Study the drawing (mm; zero at the part's minimum x, y, z) and answer. A direction names the side the tool comes from. Round coordinates to 2 decimals unless told otherwise and drop trailing zeros. Write each loop counter-clockwise with the first axis right and the second up, starting at its lowest first coordinate (ties: lowest second). Pieces come first, ordered by that corner, then holes. Notation, with made-up numbers: (-30, 73) -> (-5, 73) arc R18 cw to (-5, 108) -> close; hole circle Ø7 at (22.25, -30.75). An arc over 180 degrees is marked (long way). Return JSON: item names as keys, results as strings.
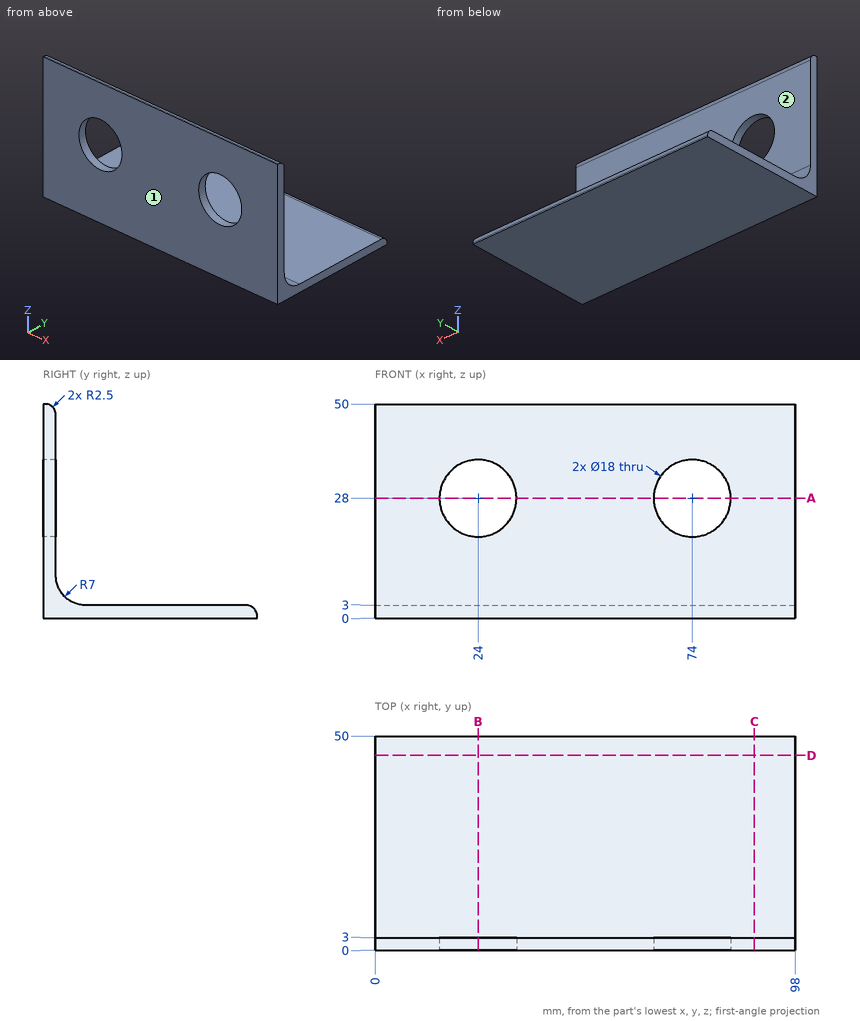
Item 1: Section D-D (y = 45.5) is taken. Give the vertices of the cut face in (x, z), then the cut area to 3 significant figures.
Worked answers:
{"outline": "(0, 0) -> (98, 0) -> (98, 3) -> (0, 3) -> close", "area": "294 mm2"}
Item 2: A tool of negligible diameter and unlimited length cuts with its end or side. For the marked faces 1 and 2, from which of +Z, -Z, +X, -X, +Y, -Y can it reach the whole face along a straight path? Write none if from no direction.
Worked answers:
{"face 1": "+Z, -Z, +X, -X, -Y", "face 2": "+Z, +X, -X, +Y"}
Item 3: Straight lines are drawn through the part: L1, parallel to Y at x = 88, z = 38.5; L2, parallel to Z at x = 74, y = 1.5. For each, find the intervals that lie inside material, in ascending order. Write a range as [from, to].
Worked answers:
{"L1": "y = [0, 3]", "L2": "z = [0, 19], [37, 49.79]"}
Item 4: Section B-B (x = 24) is taken. Give the vertices of the cut face in (y, z).
Worked answers:
{"outline": "(0, 0) -> (50, 0) -> (50, 0.5) arc R2.5 ccw to (47.5, 3) -> (10, 3) arc R7 cw to (3, 10) -> (3, 19) -> (0, 19) -> close; (0, 37) -> (3, 37) -> (3, 47.5) arc R2.5 ccw to (0.5, 50) -> (0, 50) -> close"}
Item 5: Section C-C (x = 88.5) is taken. Give the vertices of the cut face in (y, z).
Worked answers:
{"outline": "(0, 0) -> (50, 0) -> (50, 0.5) arc R2.5 ccw to (47.5, 3) -> (10, 3) arc R7 cw to (3, 10) -> (3, 47.5) arc R2.5 ccw to (0.5, 50) -> (0, 50) -> close"}
Item 6: Section A-A (z = 28) is taken. Give the vertices of the cut face in (x, y).
Worked answers:
{"outline": "(0, 0) -> (15, 0) -> (15, 3) -> (0, 3) -> close; (33, 0) -> (65, 0) -> (65, 3) -> (33, 3) -> close; (83, 0) -> (98, 0) -> (98, 3) -> (83, 3) -> close"}
Item 7: Flat-ended cylindrical pins translate along their axes: pin 1 (4 mm diameter, centred on x = 65.5, z = 22, fed in from +Y); pin 2 (10 mm diameter, centred on x = 31.5, y = 36, fed in from +Z). Find the tip coordinate at first contact, or state that the pin passes through.
Worked answers:
{"pin 1": "stops at y = 3", "pin 2": "stops at z = 3"}
